Build history of the part. All positions in model axes, mm. Face numbers are marked on the shaded views. Round coordinates to 2 decimals unless told otherwise and drop trailing zeros. Write each loop counter-clockwise with the first axis right and the second up, starting at its lowest first coordinate (ties: lowest second). Pieces come first, ordered by that corner, then holes. Notation, with made-up numbers: (-36, 34.5) -> (20, 34.5) arc R24 cw to (20, 60.5) -> close; hole circle Ø5 at (30.5, 3.5). An arc over 180 degrees is marked (long way). Return JSON: item names as keys, results as strings.
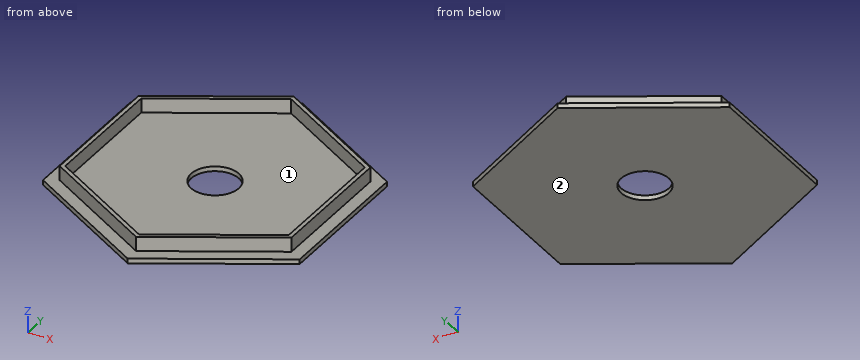
from build123d import *

# Parameters (mm, degrees)
PAD_DEPTH    = 1
PAD001_DEPTH = 3
SKETCH002_R  = 4.991419
POCKET_DEPTH = 5


with BuildPart() as part:
    # Sketch → Pad (new body)
    with BuildSketch(Plane.XY):
        Polygon((0, -31), (26.846788, -15.5), (26.846788, 15.5), (0, 31), (-26.846788, 15.5), (-26.846788, -15.5), align=None)
    extrude(amount=PAD_DEPTH)

    # Sketch001 (on Face8 of Pad) → Pad001 (join)
    with BuildSketch(Plane.XY.offset(1)):
        Polygon((0, -28), (24.248711, -14), (24.248711, 14), (0, 28), (-24.248711, 14), (-24.248711, -14), align=None)
        Polygon((0, -27), (23.382686, -13.5), (23.382686, 13.5), (0, 27), (-23.382686, 13.5), (-23.382686, -13.5), align=None, mode=Mode.SUBTRACT)
    extrude(amount=PAD001_DEPTH)

    # Sketch002 (on Face22 of Pad001) → Pocket (cut)
    with BuildSketch(Plane.XY.offset(1)):
        Circle(SKETCH002_R)
    extrude(amount=-POCKET_DEPTH, mode=Mode.SUBTRACT)


solid = part.part
Q1. Saw through at C-C on y = -10. List the corners of the cut face in (x, z).
Verdict:
{"outline": "(-26.85, 0) -> (26.85, 0) -> (26.85, 1) -> (24.25, 1) -> (24.25, 4) -> (23.38, 4) -> (23.38, 1) -> (-23.38, 1) -> (-23.38, 4) -> (-24.25, 4) -> (-24.25, 1) -> (-26.85, 1) -> close"}
Q2. Wall check: L1, parallel to Y at x = 0, z = 0.5; L2, parallel to X at y = 7, z = 2.05; L3, parallel to Z at x = -24.5, y = -7. Give the ranges that are in metal, low to high.
Verdict:
{"L1": "y = -31 to -4.99, 4.99 to 31", "L2": "x = -24.25 to -23.38, 23.38 to 24.25", "L3": "z = 0 to 1"}
Q3. Two-plate mould, pull along X, no slides. Class the marked faces 1 and 2: +X half, -X half, draft (parallel to the pull), parting line (faces both ways), or undercut.
Verdict:
{"face 1": "undercut", "face 2": "draft"}
Q4. Pin check, flat tips, straight feed: pin 1 Ø0.9 at (y, z) = (4, 2) entering from +X; pin 2 Ø4 at (x, y) = (2, 21) entering from +Z. Stop position of each tip, or through.
Verdict:
{"pin 1": "stops at x = 24.25", "pin 2": "stops at z = 1"}
Q5. Saw through at B-B on x = 1.5. List the corners of the cut face in (y, z), then the cut area to 3 significant figures.
Verdict:
{"outline": "(-30.13, 0) -> (-4.76, 0) -> (-4.76, 1) -> (-26.13, 1) -> (-26.13, 4) -> (-27.13, 4) -> (-27.13, 1) -> (-30.13, 1) -> close; (4.76, 0) -> (30.13, 0) -> (30.13, 1) -> (27.13, 1) -> (27.13, 4) -> (26.13, 4) -> (26.13, 1) -> (4.76, 1) -> close", "area": "56.7 mm²"}
Q6. Saw through at A-A on y = 0. List the corners of the cut face in (x, z).
Verdict:
{"outline": "(-26.85, 0) -> (-4.99, 0) -> (-4.99, 1) -> (-23.38, 1) -> (-23.38, 4) -> (-24.25, 4) -> (-24.25, 1) -> (-26.85, 1) -> close; (4.99, 0) -> (26.85, 0) -> (26.85, 1) -> (24.25, 1) -> (24.25, 4) -> (23.38, 4) -> (23.38, 1) -> (4.99, 1) -> close"}
Q7. Saw through at D-D on x = 13.5. List the corners of the cut face in (y, z), then the cut area to 3 significant figures.
Verdict:
{"outline": "(-23.21, 0) -> (23.21, 0) -> (23.21, 1) -> (20.21, 1) -> (20.21, 4) -> (19.21, 4) -> (19.21, 1) -> (-19.21, 1) -> (-19.21, 4) -> (-20.21, 4) -> (-20.21, 1) -> (-23.21, 1) -> close", "area": "52.4 mm²"}
